Check sheet for the drawn part. Datum: minimum x, y, z corner. Units: mm. A direction names the side the tool comes from. Round coordinates to 2 decimals unless told otherwise and drop trailing zeros. Loops run counter-clockwise (first coordinate to the right, second up) from the corner with the lowest first, then second, coordinate; pieces in that order, holes last. Notation, with made-up numbers: (4.5, 63.25) -> (21.5, 63.25) arc R12 ccw to (21.5, 73.25) -> close; hole circle Ø2 at (-23.5, 49). An arc over 180 degrees is marked (long way). Return JSON: item names as keys, results as strings.
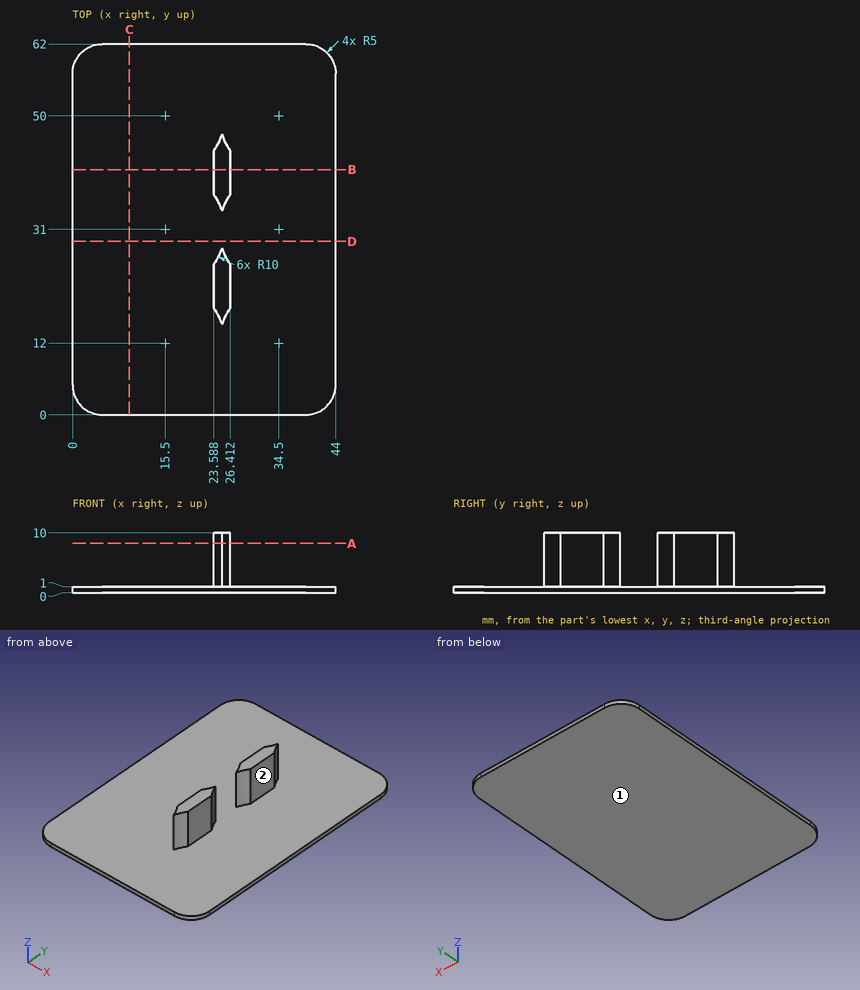
Q1. Material ranges on line 1 (Z direction, x = 33.5, y = 56); line 2 (X direction, y = 44, z = 8.5); line 3 (X direction, y = 16, z = 6.75) (1 decimal), recorded low to high.
Results list:
{"line 1": "0 to 1", "line 2": "23.59 to 26.41", "line 3": "24.7 to 25.3"}
Q2. Section check D-D (y = 29). Record the boundary of the cut face in (x, z), then the cut area to 3 significant figures.
Results list:
{"outline": "(0, 0) -> (44, 0) -> (44, 1) -> (0, 1) -> close", "area": "44.0 mm^2"}
Q3. Section check A-A (z = 8.25). Record the boundary of the cut face in (x, y).
Results list:
{"outline": "(23.59, 17.88) arc R10 cw to (25, 15.12) arc R10 cw to (26.41, 17.88) -> (26.41, 25.12) arc R10 cw to (25, 27.88) arc R10 cw to (23.59, 25.12) -> close; (23.59, 36.88) arc R10 cw to (25, 34.12) arc R10 cw to (26.41, 36.88) -> (26.41, 44.12) arc R10 cw to (25, 46.88) arc R10 cw to (23.59, 44.12) -> close"}
Q4. Tool access check on the marked faces 1 and 2. Record the directions out of +Z, -Z, +X, -X, +Y, -Y that give a thin tool (end or side, any length) a straight path to the whole face; none if there is none.
Results list:
{"face 1": "-Z, +X, -X, +Y, -Y", "face 2": "+Z, +X, +Y, -Y"}
Q5. Go/stop test with flat-tipped pins: pin 1 (3.5 mm diameter, centred on y = 40, z = 7.5, fed in from -X); pin 2 (6 mm diameter, centred on y = 40, z = 6.5, fed in from +X); pin 3 (10 mm diameter, centred on x = 7.5, y = 16.5, fed in from +Z). Record where each tip stops, or that it passes through.
Results list:
{"pin 1": "x = 23.59", "pin 2": "x = 26.41", "pin 3": "z = 1"}
Q6. Section check C-C (x = 9.5). Record the boundary of the cut face in (y, z), then the cut area to 3 significant figures.
Results list:
{"outline": "(0, 0) -> (62, 0) -> (62, 1) -> (0, 1) -> close", "area": "62.0 mm^2"}
Q7. Section check B-B (y = 41). Record the boundary of the cut face in (x, z), then the cut area to 3 significant figures.
Results list:
{"outline": "(0, 0) -> (44, 0) -> (44, 1) -> (26.41, 1) -> (26.41, 10) -> (23.59, 10) -> (23.59, 1) -> (0, 1) -> close", "area": "69.4 mm^2"}
